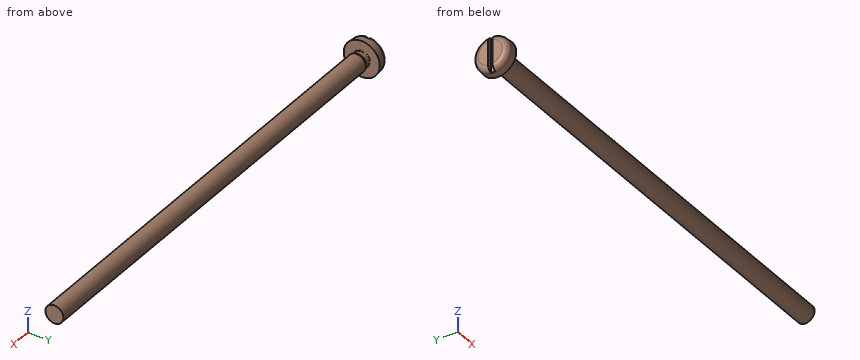
Autodesk Inventor part; units mm, degrees
ref_plane "Work Plane1" through (30.1625, 0, 0) normal (0, 0, -1) x (1, 0, 0)
ref_plane "YZ Plane" through (0, 0, 0) normal (1, 0, 0) x (0, 1, 0)
ref_plane "XZ Plane" through (0, 0, 0) normal (0, 1, 0) x (-1, 0, 0)
sketch "Sketch1" plane through (0, 0, 0) normal (0, 0, 1) x (1, 0, 0)
  line L0 (-1.3, 0) -> (20, 0)
  line L1 (20, 0) -> (20, 1)
  line L2 (20, 1) -> (0.8, 1)
  line L3 (0.8, 1) -> (0.5545, 0.8772)
  line L4 (0.5545, 0.8772) -> (0, 0.8772)
  line L5 (0, 0.8772) -> (0, 2)
  line L6 (-5.56, 0) -> (24.26, 0)
  line L7 (0, -0.4) -> (0, 2.4)
  line L8 (-1.3, 0) -> (-1.3, 1.8863)
  line L9 (0, 2) -> (-1.3, 1.8863)
  line L10 (0.8, 1) -> (0, 1) construction
  dimension "d0" = 20
  dimension "d1" = 19.2
  dimension "d2" = 0.2455
  dimension "d3" = 1.3
  dimension "d4" = 2
  dimension "d5" = 1.7545
  dimension "d9" = 4
  dimension "d10" = 5
revolve "Body" add sketch "Sketch1" angle 360 about axis through (-1.3, 0, 0) along (1, 0, 0)
sketch "Sketch2" plane through (-1.3, 0, 0) normal (-1, 0, 0) x (0, 0, 1)
  circle A0 centre (0, 0) radius 2
  line L0 (0, 0) -> (0, 1.8863)
  line L1 (-2, 0.25) -> (2, 0.25)
  line L2 (2, 0.25) -> (2, -0.25)
  line L3 (2, -0.25) -> (-2, -0.25)
  line L4 (-2, -0.25) -> (-2, 0.25)
  line L5 (-2, 0) -> (2, 0) construction
  line L6 (0, 0.25) -> (0, -0.25) construction
  dimension "d11" = 0.5
  dimension "d12" = 4
fillet "Fillet1" radius 0.6 1 edges at (-1.3, -1.8863, 0)
thread "Thread"
extrude "Slot" cut sketch "Sketch2" against normal blind 0.5 contours A0 L3 L1 | L2 L3 A0 | A0 L1 L2 | A0 L4 L1 | L3 L4 A0
ref_plane "Work Plane1" through (30.1625, 0, 0) normal (0, 0, -1) x (1, 0, 0)
fillet "Fillet5" radius 0.1 1 edges at (0, -0.8772, 0)
sketch "Sketch4" plane through (20, 0, 0) normal (1, 0, 0) x (0, 0, -1)
  circle A0 centre (0, 0) radius 1
  dimension "d42" = 2
extrude "Extrusion4" add sketch "Sketch4" along normal blind 30
thread "Thread3"
equation "\"d11\" = SBR"
equation "\"d12\" = KOD"
equation "\"d14\" = RR"
equation "\"d15\" = GEL"
equation "\"d19\" = STI"
equation "\"d41\" = R"
equation "\"d0\" = NLG"
equation "\"d1\" = GEL"
equation "\"d3\" = KOH"
equation "\"d4\" = GD"
equation "\"d5\" = BDM"
equation "\"d9\" = KOD"
equation "\"d10\" = KEWI"
equation "\"GD\" = NND"
equation "\"NLG\" = 20"
equation "\"GEL\" = 19.2"
equation "\"KOD\" = 4"
equation "\"KOH\" = 1.3"
equation "\"GAL\" = 0.61345 * PTC"
equation "\"R\" = 0.1"
equation "\"BDM\" = 1.7545"
equation "\"GUL\" = 0.61345 * PTC"
equation "\"RR\" = 0.6"
equation "\"SBR\" = 0.5"
equation "\"STI\" = 0.5"
equation "\"KEWI\" = 5deg"
equation "\"PTC\" = 0.4"
equation "\"THREADDIA\" = 2"
equation "\"TOA\" = 30deg"
equation "\"NND\" = 2"
equation "\"GD1\" = THREADDIA - 1.2269 * PTC"
properties part number "ISO 1580 - M2 x 20" material "Steel, Mild"
Geometry check sheet. Reference: the model listing, model coordinates, mm. Round coordinates to 2 decimals unless told otherwise and drop trailing zeros. Loops run counter-clockwise (first coordinate to the right, second up) from the corner with the lowest first, then second, coordinate; pieces in that order, holes last. Notation, with made-up numbers: (5, 52.25) - (43, 52.25) arc R22 cw to (43, 80.25) - close; hole circle Ø10 at (-23.75, 72). An arc over 180 degrees is marked (long way). Use a Markdown table: item, result.
Q1. Go/stop test with flat-tipped pins: P1, Ø1.5, axis at x = 28.5, y = -1.5, coming from the +Z side; P2, Ø2, axis at x = 34, z = -1.5, coming from the -Y side; P3, Ø0.6, axis at x = -1, z = -0.5, coming from the +Y side. Record where each tip stops, or that it passes through.
Solutions:
| item | result |
|---|---|
| P1 | stops at z = 0.66 |
| P2 | stops at y = -0.87 |
| P3 | stops at y = 1.91 |
Q2. Cross-section at A-A on x = 41.5. Record the cut outline in (y, z), plus the area to 3 significant figures.
Solutions:
| item | result |
|---|---|
| outline | circle Ø2 at (0, 0) |
| area | 3.14 mm2 |
Q3. Material ranges on line 1 (X direction, y = -0.45, z = 1.1); line 2 (Y direction, x = 29, z = 0); line 3 (X direction, y = 0.2, z = 0.55), recorded low to high.
Solutions:
| item | result |
|---|---|
| line 1 | x = -1.3 to 0 |
| line 2 | y = -1 to 1 |
| line 3 | x = -0.8 to 50 |
